```python
from build123d import *

# Parameters (mm, degrees)
CHAMFER1_SIZE      = 3.81
HOLE2_D            = 6
CIRPATTERN2_COUNT  = 10
HOLE4_D            = 8
CIRPATTERN4_COUNT  = 12
CUT_EXTRUDE3_REACH = 116.288
CIRPATTERN5_COUNT  = 12


with BuildPart() as part:
    # Sketch1 → Revolve1 (revolve)
    with BuildSketch(Plane.XY):
        Polygon((79.375, 10.68578), (79.375, 17.03578), (13.52042, 17.03578), (13.52042, 25.13076), (9.71042, 25.13076), (9.71042, 0), (14.14526, -4.43484), (19.22526, -4.43484), (19.22526, 10.68578), align=None)
    revolve(axis=Axis((0, 0, 0), (0, 1, 0)))

    # Chamfer1
    chamfer1_edges = [part.edges().sort_by_distance(p)[0] for p in [
        (-13.52042, 25.13076, 0),
    ]]
    chamfer(chamfer1_edges, length=CHAMFER1_SIZE - 0.0001)  # a hair under: the kernel refuses the full size

    # Hole2 (through all)
    with Locations(Plane(origin=(0, 17.03578, 0), x_dir=(1, 0, 0), z_dir=(0, 1, 0))):
        with Locations((38.1, 0)):
            hole2 = Hole(HOLE2_D / 2)

    # CirPattern2: Hole2 ×10 about axis
    cirpattern2_axis = Axis((0, 0, 0), (0, 1, 0))
    for i in range(1, CIRPATTERN2_COUNT):
        add(hole2.rotate(cirpattern2_axis, i * 360 / CIRPATTERN2_COUNT), mode=Mode.SUBTRACT)

    # Hole4 (through all)
    with Locations(Plane.XZ.offset(-10.68578)):
        with Locations((72.39, 0)):
            hole4 = Hole(HOLE4_D / 2)

    # CirPattern4: Hole4 ×12 about axis
    cirpattern4_axis = Axis((0, 0, 0), (0, 1, 0))
    for i in range(1, CIRPATTERN4_COUNT):
        add(hole4.rotate(cirpattern4_axis, i * 360 / CIRPATTERN4_COUNT), mode=Mode.SUBTRACT)

    # Sketch17 → Cut-Extrude3 (cut, up to next)
    with BuildSketch(Plane(origin=(0, 17.03578, 0), x_dir=(1, 0, 0), z_dir=(0, 1, 0)), mode=Mode.PRIVATE) as cut_extrude3_sk1:
        with BuildLine():
            ThreePointArc((79.375, 0), (77.717548697, 4.517460557), (73.531778846, 6.891049707))
            ThreePointArc((73.531778846, 6.891049707), (68.521982999, 9.388428721), (65.780227273, 14.268770092))
            ThreePointArc((65.780227273, 14.268770092), (65.016467368, 17.421109926), (64.101732931, 20.532996256))
            ThreePointArc((64.101732931, 20.532996256), (64.035992356, 26.130373726), (67.12591332, 30.798065318))
            ThreePointArc((67.12591332, 30.798065318), (69.56410177, 34.946538746), (68.740766425, 39.6875))
            ThreePointArc((68.740766425, 39.6875), (76.670362462, 20.543761705), (79.375, 0))
        make_face()
    cut_extrude3_tool1 = extrude(cut_extrude3_sk1.sketch, amount=-CUT_EXTRUDE3_REACH, mode=Mode.PRIVATE) & part.part
    cut_extrude3 = cut_extrude3_tool1.solids().sort_by_distance((71.346501, 17.03578, -19.117237))[0]
    add(cut_extrude3, mode=Mode.SUBTRACT)

    # CirPattern5: Cut-Extrude3 ×12 about axis
    cirpattern5_axis = Axis((0, 0, 0), (0, 1, 0))
    for i in range(1, CIRPATTERN5_COUNT):
        add(cut_extrude3.rotate(cirpattern5_axis, i * 360 / CIRPATTERN5_COUNT), mode=Mode.SUBTRACT)


solid = part.part
```
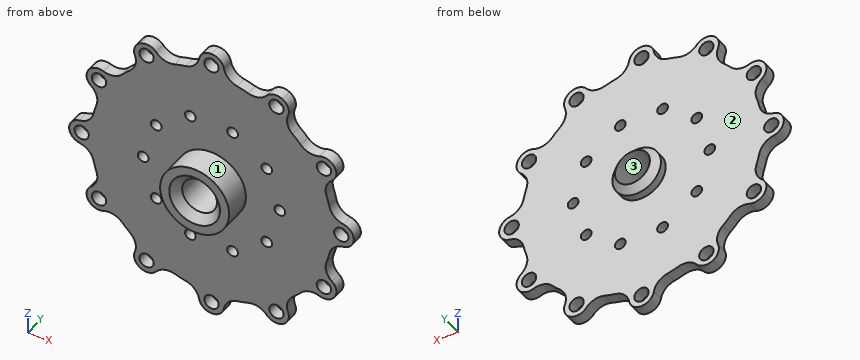
Build history of the part. All positions in model axes, mm. Face numbers are marked on the shaded views. Give positions to 0.01 mm unless a question says otherwise; leave off trailing zeros. Loops run counter-clockwise (first coordinate to the right, second up) from the corner with the lowest first, then second, coordinate; pieces in that order, holes last.
Item 1: Slice it at A-A, the plane y = 14. Give the number of separate pieces and of enclosed holes in the cut face, and give its area (3 significant figures).
Answers follow:
separate pieces: 1
enclosed holes: 23
area: 15,100 mm2
Item 2: Pull direction X, two halves, no side cores. Call the marked faces 1, 2 and 3: released by +X, released by -X, zero draft, split by the parting line, or undercut.
Answers follow:
face 1: split by the parting line
face 2: zero draft
face 3: undercut
Item 3: Drill centre lines: line 1 (Z direction, x = -36, y = 13.75); line 2 (Z direction, x = -12.5, y = 14.75); line 3 (Y direction, x = 24, z = -10). Where is each one in solid material? Low to high.
Answers follow:
line 1: z = -69.67 to -66.69, -58.7 to -2.14, 2.14 to 58.7, 66.69 to 69.67
line 2: z = -66.35 to -39.15, -33.32 to 33.32, 39.15 to 66.35
line 3: y = 10.69 to 17.04
Item 4: Slice it at B-B, the plane y = 23.25. List the corners of the cut face in (x, z).
Answers follow:
outline: circle Ø23.18 at (0, 0); hole circle Ø19.42 at (0, 0)
Item 5: Slice it at D-D, the plane y = -2. List the corners of the cut face in (x, z), and give its area (3 significant figures).
Answers follow:
outline: circle Ø38.45 at (0, 0); hole circle Ø23.42 at (0, 0)
area: 730 mm2
Item 6: Slice it at C-C, the plane z = -55.5. List the corners of the cut face in (x, y).
Answers follow:
outline: (-42.23, 10.69) - (42.23, 10.69) - (42.23, 17.04) - (-42.23, 17.04) - close
Item 7: Flat gauge pins, fed straight in: pin 1 (12 mm diameter, centred on y = 15.5, z = 16, fed in from -X); pin 2 (12 mm diameter, centred on y = 11, z = 33, fed in from +X); pin 3 (9 mm diameter, centred on x = 62.69, z = 36.2, fed in from +Y). Where does each tip first touch, or does it go through?
Answers follow:
pin 1: stops at x = -67.93
pin 2: stops at x = 69.68
pin 3: stops at y = 17.04
